Check sheet for the modelled part. Datum: model origin and axes. Units: mm. Coordinates: 2 decimals unless noted, no trailing zeros. Loops run counter-clockwise (first coordinate to the right, second up) from the corner with the lowest first, then second, coordinate; pieces in that order, holes last.
```python
from build123d import *

# Parameters (mm, degrees)
SKETCH2_W                       = 80.86
SKETCH2_H                       = 58.17
BOSS_EXTRUDE1_DEPTH             = 2.9972
F_9_64_0_14063_DIAMETER_HOLE1_D = 3.572002


with BuildPart() as part:
    # Sketch2 → Boss-Extrude1 (new body)
    with BuildSketch(Plane(origin=(0, 0, 0), x_dir=(0, 1, 0), z_dir=(0, 0, 1))):
        Rectangle(SKETCH2_W, SKETCH2_H)
    extrude(amount=BOSS_EXTRUDE1_DEPTH)

    # 9/64 (0.14063) Diameter Hole1 (through all)
    with Locations(Plane.XY.offset(2.9972)):
        with Locations((24.005, 35.35), (-24.005, -35.35)):
            Hole(F_9_64_0_14063_DIAMETER_HOLE1_D / 2)


solid = part.part
```
1) Mould release check, pull along Y, two halves, no side actions. Record for faces 1 (the flat face through (-29.085, -1, 1)), 2 (the cylindrical face through (23.045, 36.856, 1.478)), 3 (the flat face through (0, 40.43, 1)): +Y half, -Y half, draft (parallel to the pull), parting line (faces both ways), or undercut.
Answer sheet:
face 1: draft
face 2: undercut
face 3: +Y half
2) Scan lines: line 1 (Y direction, x = -23.5, z = 0.5); line 2 (Y direction, x = 23, z = 0.35). Record each from-to range of solid material in increasing order.
Answer sheet:
line 1: y = -40.43 to -37.06, -33.64 to 40.43
line 2: y = -40.43 to 33.87, 36.83 to 40.43
3) Section check A-A on y = -35.35. Enter the section's corners in (x, z) (3 decimals).
Answer sheet:
outline: (-29.085, 0) - (-25.791, 0) - (-25.791, 2.997) - (-29.085, 2.997) - close; (-22.219, 0) - (29.085, 0) - (29.085, 2.997) - (-22.219, 2.997) - close
4) Depth check by flat-ended pin: pin 1 (2 mm diameter, centred on x = 24.005, y = 35.35, fed in from +Z). Enter the tip coordinate at first touch or a pass-through.
Answer sheet:
pin 1: passes through
